from build123d import *

# Parameters (mm, degrees)
SKETCH1_R           = 60
SKETCH1_R_2         = 2.5
BOSS_EXTRUDE1_DEPTH = 4


with BuildPart() as part:
    # Sketch1 → Boss-Extrude1 (new, symmetric)
    with BuildSketch(Plane.XY):
        Circle(SKETCH1_R)
        Circle(SKETCH1_R_2, mode=Mode.SUBTRACT)
        with Locations((-10, 0)):
            Circle(SKETCH1_R_2, mode=Mode.SUBTRACT)
        with Locations((-20, 0)):
            Circle(SKETCH1_R_2, mode=Mode.SUBTRACT)
        with Locations((-30, 0)):
            Circle(SKETCH1_R_2, mode=Mode.SUBTRACT)
        with Locations((-40, 0)):
            Circle(SKETCH1_R_2, mode=Mode.SUBTRACT)
        with Locations((-50, 0)):
            Circle(SKETCH1_R_2, mode=Mode.SUBTRACT)
        with Locations((45, 0.419447228)):
            Circle(SKETCH1_R_2, mode=Mode.SUBTRACT)
        with Locations((35, 0.419447228)):
            Circle(SKETCH1_R_2, mode=Mode.SUBTRACT)
        with Locations((25, 0.419447228)):
            Circle(SKETCH1_R_2, mode=Mode.SUBTRACT)
        with Locations((15, 0.419447228)):
            Circle(SKETCH1_R_2, mode=Mode.SUBTRACT)
    extrude(amount=BOSS_EXTRUDE1_DEPTH, both=True)


solid = part.part
Read the model definition and answer for the solid it produces. Units are mm, in the model's axes. Round coordinates to 2 decimals unless told otherwise and drop trailing zeros. Write each loop counter-clockwise with the first axis right and the second up, starting at its lowest first coordinate (ties: lowest second). Pieces come first, ordered by that corner, then holes. Notation, with made-up numbers: (72, 59) - (126, 59) arc R17 ccw to (126, 65) - close; hole circle Ø7 at (-20, -17). An arc over 180 degrees is marked (long way). Use a Markdown table: item, result.
(1) The part is cut by section C-C (x = 25). Write down the section's boundary in (y, z).
Reported:
| item | result |
|---|---|
| outline | (-54.54, -4) - (-2.08, -4) - (-2.08, 4) - (-54.54, 4) - close; (2.92, -4) - (54.54, -4) - (54.54, 4) - (2.92, 4) - close |
(2) Each of these flat-tipped pins is pushed along its axis until it touches: pin 1 Ø2 at (y, z) = (24.5, 1.5) entering from +X; pin 2 Ø4 at (x, y) = (0, 0) entering from +Z; pin 3 Ø1 at (x, z) = (4.5, 3) entering from +Y; pin 4 Ø4 at (y, z) = (28, -1.5) entering from -X. Where does it stop, or does it pass through?
Reported:
| item | result |
|---|---|
| pin 1 | x = 55.21 |
| pin 2 | through |
| pin 3 | y = 59.87 |
| pin 4 | x = -54.07 |
(3) The part is cut by section A-A (x = -40). Write down the section's boundary in (y, z), then the cut area to 3 significant figures.
Reported:
| item | result |
|---|---|
| outline | (-44.72, -4) - (-2.5, -4) - (-2.5, 4) - (-44.72, 4) - close; (2.5, -4) - (44.72, -4) - (44.72, 4) - (2.5, 4) - close |
| area | 676 mm2 |
(4) The part is cut by section D-D (y = -37.5). Write down the section's boundary in (x, z).
Reported:
| item | result |
|---|---|
| outline | (-46.84, -4) - (46.84, -4) - (46.84, 4) - (-46.84, 4) - close |
(5) The part is cut by section B-B (z = -0.75). State how many separate pieces and enclosed holes the cut face has, then the cut area to 3 significant figures.
Reported:
| item | result |
|---|---|
| separate pieces | 1 |
| enclosed holes | 10 |
| area | 11,100 mm2 |
(6) The mould has two halves that part along X. Classify faces 1 (the cylindrical face through (-12.5, 0.1, -0.1)), 2 (the flat face through (12, 1, 4)), 3 (the cylindrical face through (-59.94, 2.64, 0.06)): released by +X, released by -X, zero draft, split by the parting line, or undercut.
Reported:
| item | result |
|---|---|
| face 1 | undercut |
| face 2 | zero draft |
| face 3 | split by the parting line |
(7) Straight lines are drawn through the part: line 1 along Y through (x, z) = (-30, 1.5); line 2 along Y through (x, z) = (-28.5, -3); line 3 along X through (y, z) = (31, 0.75). For each, find the intervals that lie inside material, in ascending order. Write a range as [from, to].
Reported:
| item | result |
|---|---|
| line 1 | [-51.96, -2.5], [2.5, 51.96] |
| line 2 | [-52.8, -2], [2, 52.8] |
| line 3 | [-51.37, 51.37] |
